from build123d import *

# Parameters (mm, degrees)
SKETCH1_R               = 1.5
SKETCH1_R_2             = 1
SKETCH1_W               = 12
SKETCH1_H               = 11
BOSS_EXTRUDE1_DEPTH     = 5
FILLET1_R               = 3
BOSS_EXTRUDE2_START     = -60
BOSS_EXTRUDE2_DEPTH     = 7.5
BOSS_EXTRUDE3_START     = -52.5
BOSS_EXTRUDE3_DEPTH     = 2.5
SKETCH4_R               = 2.5
SKETCH4_R_2             = 1
BOSS_EXTRUDE4_DEPTH     = 9
SKETCH5_R               = 1.5
SKETCH5_W               = 6
SKETCH5_H               = 3
CUT_EXTRUDE1_DEPTH      = 81.458933625
CUT_EXTRUDE1_DEPTH_BACK = 81.458933625
SKETCH6_W               = 10
SKETCH6_H               = 5
SKETCH6_W_2             = 5
SKETCH6_H_2             = 10
BOSS_EXTRUDE5_DEPTH     = 27
SKETCH7_W               = 40
SKETCH7_H               = 100
BOSS_EXTRUDE6_DEPTH     = 3
BOSS_EXTRUDE7_DEPTH     = 20
SKETCH9_W               = 20
SKETCH9_H               = 10
CUT_EXTRUDE2_DEPTH      = 2
BOSS_EXTRUDE8_DEPTH     = 3
SKETCH11_W              = 8
SKETCH11_H              = 15
SKETCH11_W_2            = 4
SKETCH11_H_2            = 11
BOSS_EXTRUDE9_DEPTH     = 25
SKETCH12_W              = 10
SKETCH12_H              = 7
CUT_EXTRUDE3_DEPTH      = 4


with BuildPart() as part:
    # Sketch1 → Boss-Extrude1 (new body)
    with BuildSketch(Plane(origin=(0, 0, 0), x_dir=(1, 0, 0), z_dir=(0, 1, 0))):
        Polygon((23, -32.6), (-23, -32.6), (-23, -56), (-56, -56), (-56, 23.473088065), (-43.45370132, 10.926789386), (-10.926789386, 43.45370132), (-23.473088065, 56), (23.473088065, 56), (10.926789386, 43.45370132), (43.45370132, 10.926789386), (56, 23.473088065), (56, -56), (23, -56), align=None)
        with Locations(Location((7.037702089, 20.472730932, 0), (0, 0, 270))):
            Circle(SKETCH1_R, mode=Mode.SUBTRACT)
        with Locations(Location((20.472730932, 7.037702089, 0), (0, 0, 270))):
            Circle(SKETCH1_R, mode=Mode.SUBTRACT)
        with Locations(Location((-9.5, -13.6, 0), (0, 0, 270))):
            Circle(SKETCH1_R, mode=Mode.SUBTRACT)
        with Locations(Location((9.5, -13.6, 0), (0, 0, 270))):
            Circle(SKETCH1_R, mode=Mode.SUBTRACT)
        with Locations(Location((-20.472730932, 7.037702089, 0), (0, 0, 90))):
            Circle(SKETCH1_R, mode=Mode.SUBTRACT)
        with Locations(Location((-7.037702089, 20.472730932, 0), (0, 0, 90))):
            Circle(SKETCH1_R, mode=Mode.SUBTRACT)
        with Locations(Location((29.105, -6.345, 0), (0, 0, 270))):
            Circle(SKETCH1_R_2, mode=Mode.SUBTRACT)
        with Locations(Location((49.895, -6.345, 0), (0, 0, 270))):
            Circle(SKETCH1_R_2, mode=Mode.SUBTRACT)
        with Locations(Location((49.895, -49.895, 0), (0, 0, 270))):
            Circle(SKETCH1_R_2, mode=Mode.SUBTRACT)
        with Locations(Location((29.105, -49.895, 0), (0, 0, 270))):
            Circle(SKETCH1_R_2, mode=Mode.SUBTRACT)
        Polygon((19.41207076, 27.897352134), (11.633896167, 20.119177541), (20.119177541, 11.633896167), (27.897352134, 19.41207076), align=None, mode=Mode.SUBTRACT)
        with Locations((0, -22.1)):
            Rectangle(SKETCH1_W, SKETCH1_H, mode=Mode.SUBTRACT)
        Polygon((-20.119177541, 11.633896167), (-27.897352134, 19.41207076), (-19.41207076, 27.897352134), (-11.633896167, 20.119177541), align=None, mode=Mode.SUBTRACT)
    extrude(amount=BOSS_EXTRUDE1_DEPTH)

    # Fillet1
    fillet1_edges = [part.edges().sort_by_distance(p)[0] for p in [
        (23, 2.5, 32.6),
        (-23, 2.5, 32.6),
        (-23, 2.5, 56),
        (-56, 2.5, 56),
        (-56, 2.5, -23.473088065),
        (-43.45370132, 2.5, -10.926789386),
        (-10.926789386, 2.5, -43.45370132),
        (-23.473088065, 2.5, -56),
        (23.473088065, 2.5, -56),
        (10.926789386, 2.5, -43.45370132),
        (43.45370132, 2.5, -10.926789386),
        (56, 2.5, -23.473088065),
        (56, 2.5, 56),
        (23, 2.5, 56),
    ]]
    fillet(fillet1_edges, radius=FILLET1_R)

    # Sketch3 → Boss-Extrude2 (add)
    with BuildSketch(Plane.XY.offset(56).offset(BOSS_EXTRUDE2_START)):
        with BuildLine():
            Line((-24.7, 11.72249498), (-24.7, 19.2))
            Line((-24.7, 19.2), (-51.2, 19.2))
            Line((-51.2, 19.2), (-51.2, 11.72249498))
            ThreePointArc((-51.2, 11.72249498), (-50.95, 11.1), (-51.2, 10.47750502))
            Line((-51.2, 10.47750502), (-51.2, 5))
            Line((-51.2, 5), (-49.2, 5))
            Line((-49.2, 5), (-49.2, 17.2))
            Line((-49.2, 17.2), (-26.7, 17.2))
            Line((-26.7, 17.2), (-26.7, 5))
            Line((-26.7, 5), (-24.7, 5))
            Line((-24.7, 5), (-24.7, 10.47750502))
            ThreePointArc((-24.7, 10.47750502), (-24.95, 11.1), (-24.7, 11.72249498))
        make_face()
    extrude(amount=BOSS_EXTRUDE2_DEPTH)

    # Sketch3<4> → Boss-Extrude3 (add)
    with BuildSketch(Plane.XY.offset(56).offset(BOSS_EXTRUDE3_START)):
        with BuildLine():
            Line((-21.9, 17.2), (-24.7, 17.2))
            Line((-24.7, 17.2), (-24.7, 11.72249498))
            ThreePointArc((-24.7, 11.72249498), (-23.15, 11.1), (-24.7, 10.47750502))
            Line((-24.7, 10.47750502), (-24.7, 5))
            Line((-24.7, 5), (-21.9, 5))
            Line((-21.9, 5), (-21.9, 17.2))
        make_face()
        with BuildLine():
            Line((-51.2, 11.72249498), (-51.2, 17.2))
            Line((-51.2, 17.2), (-54, 17.2))
            Line((-54, 17.2), (-54, 5))
            Line((-54, 5), (-51.2, 5))
            Line((-51.2, 5), (-51.2, 10.47750502))
            ThreePointArc((-51.2, 10.47750502), (-52.75, 11.1), (-51.2, 11.72249498))
        make_face()
    extrude(amount=-BOSS_EXTRUDE3_DEPTH)

    # Sketch4 → Boss-Extrude4 (add)
    with BuildSketch(Plane(origin=(0, 5, 0), x_dir=(1, 0, 0), z_dir=(0, 1, 0))):
        with Locations(Location((29.105, -6.345, 0), (0, 0, 270))):
            Circle(SKETCH4_R)
        with Locations(Location((29.105, -6.345, 0), (0, 0, 270))):
            Circle(SKETCH4_R_2, mode=Mode.SUBTRACT)
        with Locations(Location((29.105, -49.895, 0), (0, 0, 90))):
            Circle(SKETCH4_R)
        with Locations(Location((29.105, -49.895, 0), (0, 0, 90))):
            Circle(SKETCH4_R_2, mode=Mode.SUBTRACT)
        with Locations(Location((49.895, -49.895, 0), (0, 0, 270))):
            Circle(SKETCH4_R)
        with Locations(Location((49.895, -49.895, 0), (0, 0, 270))):
            Circle(SKETCH4_R_2, mode=Mode.SUBTRACT)
        with Locations(Location((49.895, -6.345, 0), (0, 0, 90))):
            Circle(SKETCH4_R)
        with Locations(Location((49.895, -6.345, 0), (0, 0, 90))):
            Circle(SKETCH4_R_2, mode=Mode.SUBTRACT)
    extrude(amount=BOSS_EXTRUDE4_DEPTH)

    # Sketch5 → Cut-Extrude1 (cut, two sides)
    with BuildSketch(Plane(origin=(0, 5, 0), x_dir=(1, 0, 0), z_dir=(0, 1, 0))) as cut_extrude1_sk:
        with Locations(Location((-29.5, -46, 0), (0, 0, 270))):
            Circle(SKETCH5_R)
        with Locations(Location((-49.5, -46, 0), (0, 0, 270))):
            Circle(SKETCH5_R)
        with Locations(Location((29.5, 5, 0), (0, 0, 270))):
            Circle(SKETCH5_R)
        with Locations(Location((49.5, 5, 0), (0, 0, 270))):
            Circle(SKETCH5_R)
        with Locations((-39.5, -46)):
            Rectangle(SKETCH5_W, SKETCH5_H)
        with Locations((39.5, 5)):
            Rectangle(SKETCH5_W, SKETCH5_H)
    extrude(amount=CUT_EXTRUDE1_DEPTH, mode=Mode.SUBTRACT)
    extrude(cut_extrude1_sk.sketch, amount=-CUT_EXTRUDE1_DEPTH_BACK, mode=Mode.SUBTRACT)

    # Sketch6 → Boss-Extrude5 (add)
    with BuildSketch(Plane(origin=(0, 5, 0), x_dir=(1, 0, 0), z_dir=(0, 1, 0))):
        with Locations((0, 50.5)):
            Rectangle(SKETCH6_W, SKETCH6_H)
        with Locations((-16.5, -6)):
            Rectangle(SKETCH6_W_2, SKETCH6_H_2)
        with Locations((16.5, -6)):
            Rectangle(SKETCH6_W_2, SKETCH6_H_2)
    extrude(amount=BOSS_EXTRUDE5_DEPTH)

    # Sketch7 → Boss-Extrude6 (add)
    with BuildSketch(Plane(origin=(0, 32, 0), x_dir=(1, 0, 0), z_dir=(0, 1, 0))):
        with Locations((0, 3)):
            Rectangle(SKETCH7_W, SKETCH7_H)
    extrude(amount=BOSS_EXTRUDE6_DEPTH)

    # Sketch8 → Boss-Extrude7 (add)
    with BuildSketch(Plane(origin=(0, 35, 0), x_dir=(1, 0, 0), z_dir=(0, 1, 0))):
        Polygon((-18, 51), (-18, -45), (18, -45), (18, 51), (20, 53), (20, -47), (-20, -47), (-20, 53), align=None)
    extrude(amount=BOSS_EXTRUDE7_DEPTH)

    # Sketch9 → Cut-Extrude2 (cut)
    with BuildSketch(Plane(origin=(20, 0, 0), x_dir=(0, 0, -1), z_dir=(1, 0, 0))):
        with Locations((-29, 45)):
            Rectangle(SKETCH9_W, SKETCH9_H)
    extrude(amount=-CUT_EXTRUDE2_DEPTH, mode=Mode.SUBTRACT)

    # Sketch10 → Boss-Extrude8 (add)
    with BuildSketch(Plane.XY):
        Polygon((-5.25, 5), (-5.25, 8.5), (5.25, 8.5), (5.25, 5), (4.25, 5), (4.25, 7.5), (-4.25, 7.5), (-4.25, 5), align=None)
    extrude(amount=-BOSS_EXTRUDE8_DEPTH)

    # Sketch11 → Boss-Extrude9 (add)
    with BuildSketch(Plane(origin=(0, 5, 0), x_dir=(1, 0, 0), z_dir=(0, 1, 0))):
        with Locations((21.115986736, -21.1)):
            Rectangle(SKETCH11_W, SKETCH11_H)
        with Locations((21.115986736, -21.1)):
            Rectangle(SKETCH11_W_2, SKETCH11_H_2, mode=Mode.SUBTRACT)
    extrude(amount=BOSS_EXTRUDE9_DEPTH)

    # Sketch12 → Cut-Extrude3 (cut)
    with BuildSketch(Plane.ZY.offset(-17.115986736)):
        with Locations((21.1, 8.5)):
            Rectangle(SKETCH12_W, SKETCH12_H)
    extrude(amount=-CUT_EXTRUDE3_DEPTH, mode=Mode.SUBTRACT)


solid = part.part
Geometry: final body of the model. Coordinates: model frame, mm. A direction names the side the tool comes from. Give positions to 0.01 mm unless a question says otherwise; leave off trailing zeros. Order: outer loops, then holes, each group sorted by start corner. A loop starts at its lowest first (then second) coordinate and runs counter-clockwise, first axis right, second up. Notation, with made-up numbers: (9, -7) -> (32, -7) arc R23 cw to (32, 16) -> close; hole circle Ø4 at (18, 69.5). An arc over 180 degrees is marked (long way). Put each result on its own line as item: value.
Q1. Section B-B, the plane y = 24. Return loops of the section in (x, z).
Here are the results:
outline: (-19, 1) -> (-14, 1) -> (-14, 11) -> (-19, 11) -> close; (-5, -53) -> (5, -53) -> (5, -48) -> (-5, -48) -> close; (14, 1) -> (19, 1) -> (19, 11) -> (14, 11) -> close; (17.12, 13.6) -> (25.12, 13.6) -> (25.12, 28.6) -> (17.12, 28.6) -> close; hole (19.12, 15.6) -> (23.12, 15.6) -> (23.12, 26.6) -> (19.12, 26.6) -> close
Q2. Reachability of faces 4 (the face through (27.584, 9.437, 4.361)), 5 (the face through (-38, 17.2, 0)), 6 (the face through (19, 18, 6)), 7 (the face through (0, 8, -3)) from +Z, -Z, +X, -X, +Y, -Y: full face, straight path, thin tool, end or side. Return the list, or none.
Here are the results:
face 4: +Y
face 5: +Z, -Z
face 6: -Z
face 7: +X
Q3. Draft query along Z for faces 1 (the face through (-17, 18, 1)), 2 (the face through (-19.01, 2.46, -6.71)), 3 (the face through (-17, 18, 11)). Return one class per face: released by +Z, released by -Z, zero draft, split by the parting line, or undercut.
Here are the results:
face 1: released by -Z
face 2: undercut
face 3: released by +Z
Q4. Material intervals for L1, parallel to X at y = 2, z = 46; L2, parallel to X at y = 11.1, z = 2.3; L3, parallel to X at y = 48, z = -15, sorted ascending.
Here are the results:
L1: x = -56 to -51, -48 to -42.5, -36.5 to -31, -28 to -23, 23 to 56
L2: x = -54 to -52.75, -50.95 to -49.2, -26.7 to -24.95, -23.15 to -21.9, -19 to -14, 14 to 19
L3: x = -20 to -18, 18 to 20
Q5. Section A-A, the plane z = 22.5. Return loops of the section in (x, y), then the cut area to 3 significant figures.
Here are the results:
outline: (-56, 0) -> (-6, 0) -> (-6, 5) -> (-56, 5) -> close; (-20, 32) -> (20, 32) -> (20, 40) -> (18, 40) -> (18, 35) -> (-18, 35) -> (-18, 55) -> (-20, 55) -> close; (6, 0) -> (56, 0) -> (56, 5) -> (25.12, 5) -> (25.12, 30) -> (23.12, 30) -> (23.12, 5) -> (6, 5) -> close; (17.12, 12) -> (19.12, 12) -> (19.12, 30) -> (17.12, 30) -> close; (18, 50) -> (20, 50) -> (20, 55) -> (18, 55) -> close
area: 766 mm^2
Q6. Pin query (flat end, axial travel): pin 1 (0.6 mm diameter, centred on x = 19, y = 44.5, fed in from +Z); pin 2 (22 mm diameter, centred on y = 40.5, z = 14, fed in from -X); pin 3 (1.2 mm diameter, centred on y = 6, z = -1, fed in from -X). Return the tip coordinate at first contact, or that it passes through.
Here are the results:
pin 1: stops at z = 47
pin 2: stops at x = -20
pin 3: stops at x = -51.2
Q7. Section C-C, the plane x = -29.5. Return loops of the section in (y, z).
Here are the results:
outline: (0, -24.88) -> (5, -24.88) -> (5, 44.5) -> (0, 44.5) -> close; (0, 47.5) -> (5, 47.5) -> (5, 56) -> (0, 56) -> close; (17.2, -4) -> (19.2, -4) -> (19.2, 3.5) -> (17.2, 3.5) -> close
